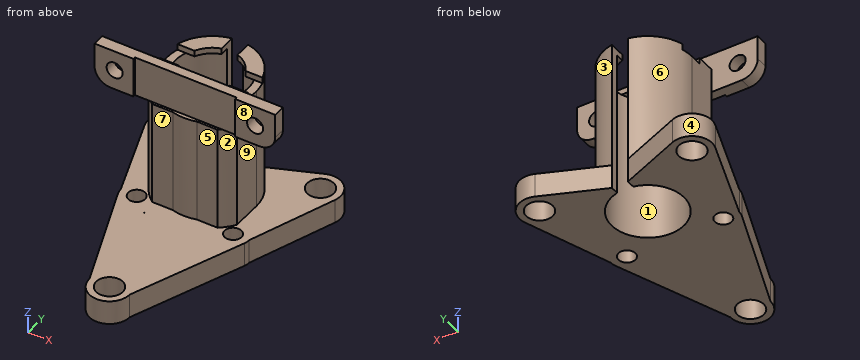
Autodesk Inventor part; units mm, degrees
ref_plane "YZ Plane" through (0, 0, 0) normal (1, 0, 0) x (0, 1, 0)
ref_plane "XZ Plane" through (0, 0, 0) normal (0, 1, 0) x (-1, 0, 0)
ref_plane "XY Plane" through (0, 0, 0) normal (0, 0, 1) x (1, 0, 0)
sketch "スケッチ1" plane through (0, 0, 0) normal (0, 0, 1) x (1, 0, 0)
  circle A0 centre (0, 0) radius 16
  line L0 (0, 0) -> (-6, 0)
  line L1 (-6, 0) -> (6, 0)
  circle A1 centre (-6, 0) radius 9
  circle A2 centre (-6, 0) radius 3
  circle A3 centre (6, 0) radius 9
  circle A4 centre (6, 0) radius 3
  circle A5 centre (-6, 0) radius 8
  circle A6 centre (0, 5.2915) radius 5
  circle A7 centre (0, 5.2915) radius 4.5
  circle A8 centre (0, 5.2915) radius 5.5
  circle A9 centre (0, 5.2915) radius 3.5
  line L2 (0, 0) -> (-11.25, 0)
  line L3 (-11.25, 0) -> (11.25, 0)
  line L4 (-11.25, 0) -> (11.25, 0)
  line L5 (11.25, 0) -> (11.25, 1.5)
  line L6 (11.25, 1.5) -> (-11.25, 1.5)
  line L7 (-11.25, 1.5) -> (-11.25, 0)
  line L8 (0, 5.2915) -> (-5.5, 5.2915)
  line L9 (0, 5.2915) -> (5.5, 5.2915)
  line L10 (5.5, 3.7915) -> (-5.5, 3.7915)
  line L11 (-5.5, 3.7915) -> (-5.5, 6.7915)
  line L12 (-5.5, 6.7915) -> (5.5, 6.7915)
  line L13 (5.5, 6.7915) -> (5.5, 3.7915)
  line L14 (5.5, 3.7915) -> (-5.5, 6.7915) construction
  line L15 (-5.5, 3.7915) -> (5.5, 6.7915) construction
  line L16 (-5.5, 5.2915) -> (-5.5, 1.5)
  line L17 (5.5, 5.2915) -> (5.5, 1.5)
  line L18 (5.2915, 3.7915) -> (5.2915, 1.5)
  line L19 (-5.2915, 3.7915) -> (-5.2915, 1.5)
  circle A10 centre (0, 5.2915) radius 6.6802
  point P0 (-3.9843, 1.5)
  point P1 (3.9843, 1.5)
  point P2 (4.0774, 0)
  point P3 (1.5, 0)
  point P4 (-4.0774, 0)
  point P5 (-1.5, 0)
  dimension "d0" = 32
  dimension "d1" = 6
  dimension "d2" = 12
  dimension "d3" = 18
  dimension "d4" = 6
  dimension "d5" = 16
  dimension "d6" = 9
  dimension "d7" = 11
  dimension "d8" = 7
  dimension "d9" = 11.25
  dimension "d10" = 22.5
  dimension "d11" = 1.5
  dimension "d12" = 3
extrude "押し出し1" add sketch "スケッチ1" along normal blind 5 contours L0 A8 A3 A6 A5 L1 | L0 A3 A8 | A8 A5 L1 | L0 A10 L6 A8 A2 | A2 A8 A3 | A8 A2 L6 A6 A3 | A5 A8 A1 L1 | A5 A6 A1 A8 | L0 L2 A2 L6 A10 | A8 L6 A2 | A6 L6 A3 | A3 L6 A7 A5 A6 | A4 A8 L6 A10 L1 | A1 A8 A4 | A5 A7 L6 A1 A6 | A1 A6 L6 A4 A8 | L2 L7 L6 A2 | A10 L6 A4 L3 L1 | A4 L6 A8 | A7 L6 A5 | A5 L6 A7 | A1 L6 A6 | A4 L6 L5 L3 picked at (2.524, 0.7859) picked at (-3.6973, 1.4091) picked at (3.6973, 1.4091)
extrude "押し出し2" add sketch "スケッチ1" along normal blind 3 contours L0 A8 A3 A6 A5 L1 | A8 A2 L6 A6 A3 | A5 A6 A1 A8 | A8 L6 A2 | A6 L6 A3 | A3 L6 A7 A5 A6 | A5 A7 L6 A1 A6 | A1 A6 L6 A4 A8 | L16 A2 L19 L6 | L6 A8 A2 | A2 A6 L6 | L6 L19 A2 A8 | L6 A6 L10 A7 A3 | A3 A7 L6 | A4 L6 A8 | A7 L6 A5 | A5 L6 A7 | A1 L6 A6 | L16 L10 L19 A2 | A2 A8 L10 A6 | A2 L19 A8 | A7 L10 A9 A3 | A3 A9 A5 L6 A7 | L6 L18 A4 L17 | L6 A6 A4 | A4 A8 L6 | A8 A4 L18 L6 | A5 A9 A1 A7 L6 | A7 A1 L6 | A1 A7 L10 A6 L6 | L11 A8 L10 | L10 A8 L8 A6 | A6 L8 A7 L10 | A8 A1 A6 A5 | A5 A6 L12 A8 | A7 L8 A9 L10 | A4 L18 L10 L17 | A6 L10 A8 A4 | A8 L18 A4 | A1 A9 L10 A7 | A8 L12 A6 L8 | A6 L12 A7 L8 | A8 A3 A6 A1 | A6 A1 A7 A5 | A5 A7 L12 A6 | A7 L12 A9 L8 | L10 A8 L13 | L10 A7 L9 A6 | A6 L9 A8 L10 | L10 A9 L9 A7 | A6 A3 A7 A1 | A8 L12 A6 A3 | A7 A1 A9 A5 | A5 A9 L12 A7 | L9 A6 L12 A8 | L9 A7 L12 A6 | L9 A9 L12 A7 | A7 A3 A9 A1 | A6 L12 A7 A3 | L12 A9 A3 A7
extrude "押し出し3" cut sketch "スケッチ1" along normal blind 2.25 contours A7 L6 A5 | A5 L6 A7 | A7 L10 A9 A3 | A3 A9 A5 L6 A7 | A5 A9 A1 A7 L6 | A7 L8 A9 L10 | A1 A9 L10 A7 | A7 L12 A9 L8 | L10 A9 L9 A7 | A7 A1 A9 A5 | A5 A9 L12 A7 | L9 A9 L12 A7 | A7 A3 A9 A1 | L12 A9 A3 A7
sketch "スケッチ2" plane through (0, 0, 3) normal (0, 0, 1) x (1, 0, 0)
  line L0 (5.5, 3.7903) -> (-5.5, 3.7903)
  line L1 (-5.5, 3.7903) -> (-5.5, 6.7903)
  line L2 (-5.5, 6.7903) -> (5.5, 6.7903)
  line L3 (5.5, 6.7903) -> (5.5, 3.7903)
  line L4 (5.5, 3.7903) -> (-5.5, 6.7903) construction
  line L5 (-5.5, 3.7903) -> (5.5, 6.7903) construction
  point P0 (0, 0)
  point P1 (0, 5.2903)
  dimension "d19" = 11
  dimension "d20" = 3
extrude "押し出し4" cut sketch "スケッチ2" against normal blind 0.75
extrude "押し出し5" add sketch "スケッチ1" against normal blind 16 contours L1 A8 L0 | L0 A8 A3 A6 A5 L1 | L0 A3 A8 | A8 A5 L1 | L0 A10 L6 A8 A2 | A2 A8 A3 | A8 A2 L6 A6 A3 | A5 A8 A1 L1 | A5 A6 A1 A8 | A8 L6 A2 | A6 L6 A3 | A3 L6 A7 A5 A6 | A4 A8 L6 A10 L1 | A1 A8 A4 | A5 A7 L6 A1 A6 | A1 A6 L6 A4 A8 | L16 A2 L19 L6 | L6 A8 A2 | A2 A6 L6 | L6 L19 A2 A8 | L6 A6 L10 A7 A3 | A3 A7 L6 | A4 L6 A8 | A1 L6 A6 | L16 L10 L19 A2 | A2 A8 L10 A6 | A2 L19 A8 | L6 L18 A4 L17 | L6 A6 A4 | A4 A8 L6 | A8 A4 L18 L6 | A7 A1 L6 | A1 A7 L10 A6 L6 | L11 A8 L10 | L10 A8 L8 A6 | A6 L8 A7 L10 | A8 A1 A6 A5 | A5 A6 L12 A8 | A4 L18 L10 L17 | A6 L10 A8 A4 | A8 L18 A4 | A8 L12 A6 L8 | A6 L12 A7 L8 | A8 A3 A6 A1 | A6 A1 A7 A5 | A5 A7 L12 A6 | L10 A8 L13 | L10 A7 L9 A6 | A6 L9 A8 L10 | A6 A3 A7 A1 | A8 L12 A6 A3 | L9 A6 L12 A8 | L9 A7 L12 A6 | A6 L12 A7 A3
sketch "電池" plane through (0, 0, -16) normal (0, 0, -1) x (-1, 0, 0)
  line L0 (0, 0) -> (0, 8)
  circle A0 centre (0, 8) radius 8
  dimension "d34" = 8
sketch "スケッチ3" plane through (0, 5.2915, -16) normal (0, 0, -1) x (-1, 0, 0)
  line L0 (0, -5.2915) -> (-6, -5.2915)
  line L1 (11.25, -5.2915) -> (-11.25, -5.2915)
  line L2 (-6, -5.2915) -> (6, -5.2915)
  circle A0 centre (-6, -5.2915) radius 3
  circle A1 centre (-6, -5.2915) radius 9
  circle A2 centre (6, -5.2915) radius 3
  circle A3 centre (6, -5.2915) radius 9
  circle A4 centre (-6, -5.2915) radius 10
  circle A5 centre (6, -5.2915) radius 10
  line L3 (0, -5.2915) -> (11, -5.2915)
  line L4 (0, -5.2915) -> (0, 6.2085)
  line L5 (0, 6.2085) -> (9.5, 6.2085)
  line L6 (9.5, 6.2085) -> (-9.5, 6.2085)
  circle A6 centre (-9.5, 6.2085) radius 1.65
  circle A7 centre (9.5, 6.2085) radius 1.65
  circle A8 centre (-9.5, 6.2085) radius 2.5
  circle A9 centre (9.5, 6.2085) radius 2.5
  circle A10 centre (6, -5.2915) radius 1.05
  circle A11 centre (-6, -5.2915) radius 1.05
  line L7 (0, -5.2915) -> (0, -6.5915)
  line L8 (-5.5, -3.7915) -> (-5.5, -1.5012)
  line L9 (0, -6.5915) -> (11.25, -6.5915)
  line L10 (11.25, -6.5915) -> (11.25, -5.2915)
  line L11 (0, -6.5915) -> (-11.25, -6.5915)
  line L12 (-11.25, -6.5915) -> (-11.25, -5.2915)
  line L13 (0, -6.5915) -> (0, -14.5915)
  line L14 (0, -14.5915) -> (11.25, -14.5915)
  line L15 (11.25, -14.5915) -> (11.25, -15.8915)
  line L16 (11.25, -15.8915) -> (-11.25, -15.8915)
  line L17 (-11.25, -15.8915) -> (-11.25, -14.5915)
  line L18 (0, -14.5915) -> (-11.25, -14.5915)
  line L19 (0, -15.8915) -> (0, -19.8915)
  circle A12 centre (0, -19.8915) radius 1.65
  circle A13 centre (0, -19.8915) radius 2.5
  line L20 (-2.5, -19.8915) -> (2.5, -19.8915)
  circle A14 centre (0, 0) radius 5.5
  circle A15 centre (-6, -5.2915) radius 2
  circle A16 centre (6, -5.2915) radius 2
  line L21 (-9.5, 3.7085) -> (9.5, 3.7085)
  line L22 (-8, -5.2915) -> (-8, 3.7085)
  line L23 (8, -5.2915) -> (8, 3.7085)
  line L24 (-6, -7.2915) -> (6, -7.2915)
  line L25 (2.5, -19.8915) -> (2.5, -7.2915)
  line L26 (-2.5, -19.8915) -> (-2.5, -7.2915)
  line L27 (1, -5.5) -> (-1, -5.5)
  line L28 (-1, -5.5) -> (-1, 5.5)
  line L29 (-1, 5.5) -> (1, 5.5)
  line L30 (1, 5.5) -> (1, -5.5)
  line L31 (1, -5.5) -> (-1, 5.5) construction
  line L32 (-1, -5.5) -> (1, 5.5) construction
  circle A17 centre (0, 0) radius 4.5
  line L33 (-1, 5.4083) -> (-8.5471, 8.5198)
  line L34 (1, 5.4083) -> (8.5471, 8.5198)
  line L35 (-8, -5.2915) -> (-11.851, 5.3584)
  line L36 (8, -5.2915) -> (11.851, 5.3584)
  line L37 (-2.5, -19.8915) -> (-7.8655, -6.0127)
  line L38 (2.5, -19.8915) -> (7.8655, -6.0127)
  point P0 (3.7639, -7.2915)
  point P1 (3.798, -7.2915)
  point P2 (3.7917, -7.3221)
  point P3 (-3.7639, -7.2915)
  point P4 (-3.7917, -7.3221)
  point P5 (-3.798, -7.2915)
  point P6 (3, -5.2915)
  point P7 (1.5, -5.2915)
  point P8 (-1.5, -5.2915)
  point P9 (-4, -5.2915)
  point P10 (-3.8997, -3.8785)
  point P11 (3.0937, -4.5474)
  point P12 (-1, -4.3875)
  point P13 (1, -4.3875)
  point P14 (1, 5.4083)
  dimension "d25" = 6
  dimension "d26" = 12
  dimension "d27" = 6
  dimension "d28" = 18
  dimension "d35" = 20
  dimension "d36" = 20
  dimension "d37" = 11
  dimension "d38" = 11.5
  dimension "d39" = 9.5
  dimension "d40" = 19
  dimension "d41" = 3.3
  dimension "d42" = 3.3
  dimension "d43" = 5
  dimension "d44" = 5
  dimension "d45" = 2.1
  dimension "d46" = 2.1
  dimension "d47" = 1.3
  dimension "d48" = 8
  dimension "d49" = 1.3
  dimension "d50" = 4
  dimension "d51" = 3.3
  dimension "d52" = 5
  dimension "d53" = 11
  dimension "d54" = 4
  dimension "d55" = 4
  dimension "d56" = 2
  dimension "d57" = 11
  dimension "d58" = 9
sketch "スケッチ4" plane through (-11.25, 0, 5) normal (0, -1, 0) x (1, 0, 0)
  line L0 (0, 0) -> (22.5, 0)
  line L1 (0, 0) -> (2.5, 0)
  line L2 (2.5, 0) -> (2.5, -2.5)
  line L3 (2.5, -2.5) -> (20, -2.5)
  circle A0 centre (2.5, -2.5) radius 1
  circle A1 centre (20, -2.5) radius 1
  line L4 (0.1664, -5) -> (4.8336, -5)
  line L5 (4.8336, -5) -> (4.8336, 0)
  line L6 (4.8336, 0) -> (0.1664, 0)
  line L7 (0.1664, 0) -> (0.1664, -5)
  line L8 (0.1664, -5) -> (4.8336, 0) construction
  line L9 (4.8336, -5) -> (0.1664, 0) construction
  line L10 (22.5, -5) -> (17.5, -5)
  line L11 (17.5, -5) -> (17.5, 0)
  line L12 (17.5, 0) -> (22.5, 0)
  line L13 (22.5, 0) -> (22.5, -5)
  line L14 (22.5, -5) -> (17.5, 0) construction
  line L15 (17.5, -5) -> (22.5, 0) construction
  line L16 (4.8336, -5) -> (17.5, -5)
  point P0 (11.25, -5)
  dimension "d29" = 2.5
  dimension "d30" = 2.5
  dimension "d31" = 17.5
  dimension "d32" = 2
  dimension "d33" = 2
  dimension "d63" = 5
  dimension "d64" = 5
extrude "押し出し6" add sketch "スケッチ3" against normal blind 3 contours A0 L11 A5 L0 | A3 L11 A0 | L0 A14 L28 L27 L7 L11 A3 | A15 L11 L1 A11 L0 | A15 L8 A0 A14 A5 | L0 A11 L1 A15 | A5 L11 A15 | L11 A3 L24 A0 | A0 L24 A5 L11 | L11 L13 L24 A3 | A5 L24 A15 L11 | A15 L22 A0 L8 | A15 L11 | A14 L27 L28 | L24 A3 L26 A5 A0 | L24 L26 A3 | L7 L27 L30 A14 L1 A1 L9 | L9 A1 L24 L13 | A0 L22 A1 A14 | A5 A0 L37 L11 A15 L24 | L35 A0 L22 | L11 L37 A15 | A14 L30 L27 | A5 L26 A1 L37 A0 | L26 L24 L13 A3 | A3 A1 A5 L26 | L9 A2 L24 A1 | A1 A2 L9 | L24 L25 A1 L13 | A1 L21 A14 | A0 L35 A1 L22 | A5 A1 L26 | L13 A5 A1 | A1 L25 A4 A3 | A3 A4 L13 | L24 A2 A4 L25 A1 | A1 L25 L24 | A2 A14 A4 L1 | L1 A4 L9 A2 | L9 A4 L24 A2 | A1 L22 L21 | L21 A8 A4 A14 | A1 L35 A4 A8 L21 L22 | A1 L26 L18 L37 | A5 A4 L18 L26 A1 | A4 L25 A3 | A3 L25 L14 A5 A4 | L13 L18 A4 | A5 L14 L13 | A16 L1 A10 | A16 L9 A4 | A4 A14 A2 L23 A16 | L1 A10 A16 L9 | L9 A16 L24 A4 | A4 A8 L6 L33 A14 | L35 A8 A4 | L18 L26 A4 L37 | L18 A4 L26 | A4 A2 L38 A3 L25 | A3 L38 L14 L25 | L18 L14 A5 L25 L16 L26 A4 | L14 L25 A5 | A4 L24 A16 L9 L38 A2 | L23 A2 L36 | L9 A16 | A8 A4 | A4 A8 | A4 L26 L16 L37 | L14 L38 A5 L25 | A5 L38 L16 L25 | A14 A3 L23 A2 | L38 L9 A16 | L23 A3 L36 A2 | A8 L33 L6 | L16 L26 L37 | L16 L19 A13 L26 | A14 L21 A3 | L25 A13 L19 L16 | L16 L38 L25 | L23 L21 A9 A5 L36 A3 | A3 L21 L23 | L34 L5 A9 A5 A14 | L20 A12 A13 | A13 L19 A12 L20 | L21 A14 A5 A9 | L20 A12 L19 A13 | A5 A9 L36 | L34 A9 L5 | A9 A5 | A5 A9
extrude "押し出し7" cut sketch "スケッチ3" against normal blind 19 contours L28 A3 L4 A17 | L28 A5 A1 A3 | L4 A1 L30 A17 | L28 A1 A5 | A3 A4 L30 A1 | L4 A4 A3 | A1 A5 L4 | A1 L28 A4 A5 | A4 A5 L30 A3 | A3 L30 A4 | L4 L21 L30 A5 | A4 L28 L21 L4 | L21 L28 A17 L4 | L4 A17 L30 L21 | A14 L4 A17 L28 | L4 A14 L30 A17
extrude "押し出し8" cut sketch "スケッチ4" against normal blind 0.3 contours L0 L11 L3 L5 | L5 L3 L11 L16
extrude "押し出し9" cut sketch "スケッチ4" against normal blind 1.5 contours A0 L3 L2 | L2 L3 A0 | A1
fillet "フィレット1" radius 2 2 edges at (-11.25, 0.75, 0) (11.25, 0.75, 0)
properties part number "ikafly2"
Input: part model. Units: mm. Frame: model coordinates. Face numbers are marked on the shaded views. A direction names the side the tool comes from. Round coordinates to 2 decimals unless told otherwise and drop trailing zeros. Loops run counter-clockwise (first coordinate to the right, second up) from the corner with the lowest first, then second, coordinate; pieces in that order, holes last. Notation, with made-up numbers: (80.5, 70.5) - (114.5, 70.5) arc R27 cw to (114.5, 109.5) - close; hole circle Ø3 at (16, -11). An arc over 180 degrees is marked (long way). One line per item, written item: value. Start each with the question number.
(1) Section A-A, the plane x = 0. Return loops of the section in (y, z), plus the area to 3 significant figures.
(2) Section B-B, the plane x = -6. Return loops of the section in (y, z).
(3) Ray query, line 1 (X direction, y = 1.1, z = 2.5); line 2 (X direction, y = 0.7, z = 2.5); line 3 (X direction, y = 12, z = -15). Return the intervals inside material, ascending. Write a range as [from, to].
(4) Access query for the marked faces 5, 6, 7, 8 and 9. Directions: +Z, -Z, +X, -X, +Y, -Y. A direction counts if a zero-diameter tool reaches every point of the face in a straight line with its end or side. Return the directions, or none.
(5) Section D-D, the plane z = -13.5. Count the separate pieces of the cut face and the enclosed holes in it, plus the area to 3 significant figures.
(6) Draft query along Y for the marked faces 1, 2, 3 and 4. Return one class per face: +Y half, -Y half, draft (parallel to the pull), parting line (faces both ways), or undercut.
(7) Section C-C, the plane y = 11.5. Return loops of the section in (x, z).
(8) Contact query for flat-ended pins moving along their axis: P1, Ø2, axis at x = 5.5, z = -6, coming from the +Y side; P2, Ø12, axis at x = -0.5, z = -13.5, coming from the +Y side; P3, Ø1.1, axis at y = 3.5, z = -8.5, coming from the +X side. Output: stop coordinate, or through.
Results below:
1. outline: (-17.1, -16) - (-16.25, -16) - (-16.25, -13) - (-17.1, -13) - close; (-12.95, -16) - (0.79, -16) - (0.79, 3) - (1.5, 3) - (1.5, 5) - (0.3, 5) - (0.3, 0) - (-0.21, 0) - (-0.21, -13) - (-12.95, -13) - close
1. area: 60.6 mm^2
2. outline: (-5.55, -16) - (-1.05, -16) - (-1.05, -13) - (-5.55, -13) - close; (0.3, 0) - (1.5, 0) - (1.5, 5) - (0.3, 5) - close; (1.05, -16) - (12.76, -16) - (12.76, -13) - (1.05, -13) - close
3. line 1: [-11.25, -9.75], [-7.75, -1], [1, 7.75], [9.75, 11.25]
3. line 2: [-11.25, -9.75], [-7.75, 7.75], [9.75, 11.25]
3. line 3: [-11.95, -11.07], [-7.93, -4.15], [4.15, 7.93], [11.07, 11.95]
4. face 5: +Z, +X, -Y
4. face 6: +Z, -X, +Y
4. face 7: +Z, -X, -Y
4. face 8: +Z, +X, -X, -Y
4. face 9: +Z, +X, +Y
5. separate pieces: 1
5. enclosed holes: 7
5. area: 323 mm^2
6. face 1: undercut
6. face 2: -Y half
6. face 3: +Y half
6. face 4: parting line
7. outline: (-12, -16) - (-11.15, -16) - (-11.15, -13) - (-12, -13) - close; (-7.85, -16) - (-2.94, -16) - (-2.94, -13) - (-7.85, -13) - close; (2.94, -16) - (7.85, -16) - (7.85, -13) - (2.94, -13) - close; (11.15, -16) - (12, -16) - (12, -13) - (11.15, -13) - close
8. P1: y = 8.45
8. P2: y = 12.97
8. P3: x = 5.5
